Work out the finished part from the listing and answer in its coordinate system (mm). A direction names the side the tool comes from. Round coordinates to 2 decimals unless told otherwise and drop trailing zeros. Loops run counter-clockwise (first coordinate to the right, second up) from the corner with the lowest first, then second, coordinate; pieces in that order, holes last. Notation, with made-up numbers: (84, 53.5) -> (111, 53.5) arc R32 cw to (111, 79.5) -> close; hole circle Ø11 at (-36.5, 4). An arc over 180 degrees is marked (long way). Write item = value, one per line. Start each with the question number.
```python
from build123d import *

# Parameters (mm, degrees)
F0_R     = 0.5
F1_DEPTH = 3
F2_W     = 3
F2_H     = 6
F3_DEPTH = 6


with BuildPart() as f1:
    # F0 (on Top) → F1 (new body)
    with BuildSketch(Plane.XY):
        Polygon((0, 6), (0, 0), (6, 0), (6, 6), (4, 6), align=None)
        with Locations((4, 3)):
            Circle(F0_R, mode=Mode.SUBTRACT)
    extrude(amount=F1_DEPTH)

    # F2 (on Top) → F3 (join)
    with BuildSketch(Plane.XY):
        with Locations((1.5, 3)):
            Rectangle(F2_W, F2_H)
    extrude(amount=F3_DEPTH)


solid = f1.part
```
Item 1: Flat-ended cylindrical pins translate along their axes: pin 1 (1.5 mm diameter, centred on x = 4.5, y = 3.5, fed in from +Z); pin 2 (2.5 mm diameter, centred on y = 2.5, z = 4.5, fed in from +X). Find the tip coordinate at first contact, or state that the pin passes through.
Item 2: Section A-A (x = 4) is taken. Determine the outline of the cut face in (y, z), then the cut area to 3 significant figures.
Item 3: Section B-B (y = 3) is taken. Determine the outline of the cut face in (x, z), then the cut area to 3 significant figures.
Item 4: Section C-C (z = 1.55) is taken. Determine the outline of the cut face in (x, y), then the cut area to 3 significant figures.
Item 5: The mould has two halves that part along Y. Classify faces 3 (the flat face through (6, 3, 1)), 4 (the cylindrical face through (3.935, 3.496, 1.479)), 5 (the flat face through (2, 0, 2)): pulls with the +Y half, pulls with the -Y half, needs draft (parallel to the pull), parting line crosses it, or undercut.
Item 6: Find the intervals of material crossed by line 1 along Y through (x, z) = (4, 0.6); line 2 along X through (y, z) = (4.2, 3.95), in increasing order. Write a range as [from, to].
Item 7: A tool of negligible diameter and unlimited length cuts with its end or side. For faces 1 (the flat face through (1, 3, 6)), 2 (the flat face through (5, 3, 3)), from which of +Z, -Z, +X, -X, +Y, -Y can it reach the whole face along a straight path? Write none if from no direction.
Item 8: Section D-D (y = 1.85) is taken. Determine the outline of the cut face in (x, z), then the cut area to 3 significant figures.
Worked answers:
q1.pin_1 = 3
q1.pin_2 = 3
q2.outline = (0, 0) -> (2.5, 0) -> (2.5, 3) -> (0, 3) -> close; (3.5, 0) -> (6, 0) -> (6, 3) -> (3.5, 3) -> close
q2.area = 15.0 mm2
q3.outline = (0, 0) -> (3.5, 0) -> (3.5, 3) -> (3, 3) -> (3, 6) -> (0, 6) -> close; (4.5, 0) -> (6, 0) -> (6, 3) -> (4.5, 3) -> close
q3.area = 24.0 mm2
q4.outline = (0, 0) -> (6, 0) -> (6, 6) -> (0, 6) -> close; hole circle Ø1 at (4, 3)
q4.area = 35.2 mm2
q5.face_3 = needs draft
q5.face_4 = undercut
q5.face_5 = pulls with the -Y half
q6.line_1 = [0, 2.5], [3.5, 6]
q6.line_2 = [0, 3]
q7.face_1 = +Z, +X, -X, +Y, -Y
q7.face_2 = +Z, +X, +Y, -Y
q8.outline = (0, 0) -> (6, 0) -> (6, 3) -> (3, 3) -> (3, 6) -> (0, 6) -> close
q8.area = 27.0 mm2
